Could you check a few things on this model? Use its own coordinates, in mm. A direction names the side the tool comes from. Coordinates: 2 decimals unless noted, no trailing zeros. Loops run counter-clockwise (first coordinate to the right, second up) from the corner with the lowest first, then second, coordinate; pieces in that order, holes last. Notation, with made-up numbers: M 31.5,31 L 73.5,31 A10 ccw 73.5,39 Z; hole C 8.25,61.25 d2. An arc over 180 degrees is marked long. Write each question's results on one line, items separated by ' | '.
```python
from build123d import *

# Parameters (mm, degrees)
STOCK_TEST_FINGER_MICHELLE_V2_1_START = -21.07817965
STOCK_TEST_FINGER_MICHELLE_V2_1_DEPTH = 2.5
CUT_EXTRUDE1_START                    = -1.5
SKETCH1_R                             = 1.75
CUT_EXTRUDE1_DEPTH                    = 1.5
SKETCH2_W                             = 20.99
SKETCH2_H                             = 12.7
CUT_EXTRUDE2_DEPTH                    = 23.542331171


# Read off the part's stored shape, not the designer's step: Stock-test_finger_michelle_V2-1
with BuildPart() as part:
    # Stock-test_finger_michelle_V2-1 outline → Stock-test_finger_michelle_V2-1 (new body)
    with BuildSketch(Plane.YZ.offset(STOCK_TEST_FINGER_MICHELLE_V2_1_START)):
        Polygon((0, -6.34419618), (9.2, -15.54419618), (12.7, -15.54419618), (12.7, 18.45580382), (9.2, 18.45580382), (0, 9.25580382), align=None)
    extrude(amount=STOCK_TEST_FINGER_MICHELLE_V2_1_DEPTH)

    # Sketch1 → Cut-Extrude1 (cut)
    with BuildSketch(Plane.ZY.offset(21.07817965).offset(CUT_EXTRUDE1_START)):
        with Locations(Location((-12.29419618, 9.2, 0), (0, 0, 180))):
            Circle(SKETCH1_R)
        with Locations(Location((15.20580382, 9.2, 0), (0, 0, 180))):
            Circle(SKETCH1_R)
    extrude(amount=CUT_EXTRUDE1_DEPTH, mode=Mode.SUBTRACT)

    # Sketch2 → Cut-Extrude2 (cut, through all)
    with BuildSketch(Plane.ZY.offset(21.07817965)):
        with Locations((-5.04919618, 6.35)):
            Rectangle(SKETCH2_W, SKETCH2_H)
    extrude(amount=-CUT_EXTRUDE2_DEPTH, mode=Mode.SUBTRACT)

    # Mirror1: part across plane


with BuildPart() as part_1:
    add(part.part)
    add(part.part.mirror(Plane(origin=(0, 0, 5.44580382), x_dir=(1, 0, 0), z_dir=(0, 0, -1))))


solid = part_1.part
```
(1) Imagine slicing it at A-A, the plane x = -19.9. List the corners of the cut face in (y, z) for me.
Reported:
outline: M 0,1.64 L 9.2,-7.56 L 12.7,-7.56 L 12.7,18.46 L 9.2,18.46 L 0,9.26 Z; hole C 9.2,-4.31 d3.5; hole C 9.2,15.21 d3.5
(2) Please list where these lines run through material, in increasing order: probe 1 along Z at (x, y) = (-20.05, 9.5); probe 2 along Z at (x, y) = (-20.1, 8.5); probe 3 along Y at (x, z) = (-20.45, 16.5). Write a range as from..to.
Reported:
probe 1: z = -7.56..-6.04, -2.59..13.48, 16.93..18.46 | probe 2: z = -6.86..-5.92, -2.71..13.6, 16.81..17.76 | probe 3: y = 7.24..8.02, 10.38..12.7
(3) Will these pins go through, and if not, where does the flat tip stop? P1, Ø3, axis at y = 9.2, z = -4.31, coming from the -X side; P2, Ø4, axis at y = 9, z = 14.5, coming from the -X side.
Reported:
P1: stops at x = -19.58 | P2: stops at x = -21.08
(4) Imagine slicing it at B-B, the plane z = 14.25. List the corners of the cut face in (x, y) for me, and give its area (3 significant figures).
Reported:
outline: M -21.08,4.99 L -18.58,4.99 L -18.58,12.7 L -21.08,12.7 L -21.08,10.67 L -19.58,10.67 L -19.58,7.73 L -21.08,7.73 Z | area: 14.9 mm2
(5) Which directions (+Z, -Z, +X, -X, +Y, -Y) give clear straight access to the entire face, cutting with the end or side of a thin tool? Please do faces 4 (the flat face through (-18.578, 8, 5)), 5 (the flat face through (-19.578, 9, -4)).
Reported:
face 4: +Z, -Z, +X, +Y, -Y | face 5: -X
(6) If we mould it in two halves opening along Z, with no side actions, what happens to faces 1 (the flat face through (-20, 0, 5)), 2 (the cylindrical face through (-20.32, 8.02, 16.5)), 3 (the flat face through (-20, 11, 18.456))? For each: released by +Z, released by -Z, zero draft, split by the parting line, or undercut.
Reported:
face 1: zero draft | face 2: undercut | face 3: released by +Z
(7) Imagine slicing it at C-C, the plane y = 9.75. List the corners of the cut face in (x, z) for me.
Reported:
outline: M -21.08,-7.56 L -18.58,-7.56 L -18.58,18.46 L -21.08,18.46 L -21.08,16.87 L -19.58,16.87 L -19.58,13.54 L -21.08,13.54 L -21.08,-2.65 L -19.58,-2.65 L -19.58,-5.98 L -21.08,-5.98 Z
(8) Imagine slicing it at D-D, the plane z = -4.75. List the corners of the cut face in (x, y) for me, and give its area (3 significant figures).
Reported:
outline: M -21.08,6.39 L -18.58,6.39 L -18.58,12.7 L -21.08,12.7 L -21.08,10.89 L -19.58,10.89 L -19.58,7.51 L -21.08,7.51 Z | area: 10.7 mm2
